Source: CAD feature listing. Evaluate the final solid. Frame: model axes, mm. A direction names the side the tool comes from. Round coordinates to 2 decimals unless told otherwise and drop trailing zeros. Order: outer loops, then holes, each group sorted by start corner. A loop starts at its lowest first (then second) coordinate and runs counter-clockwise, first axis right, second up. Notation, with made-up numbers: M 55.25,-4.75 L 100.25,-4.75 A25 ccw 100.25,34.25 Z; hole C 42.25,27.25 d10. An arc over 180 degrees is marked long. Use CSV: the item, a comma, the result in double quotes. Start each with the question number.
```python
from build123d import *

# Parameters (mm, degrees)
IZIM1_R                     = 2.35
IZIM1_R_2                   = 0.5
Y_KSEKLIK_EKSTR_ZYON1_DEPTH = 1.5
IZIM1_3_R                   = 2.35
IZIM1_3_R_2                 = 1.275
Y_KSEKLIK_EKSTR_ZYON2_DEPTH = 0.5
IZIM2_R                     = 3.45
IZIM2_R_2                   = 2.3
Y_KSEKLIK_EKSTR_ZYON3_DEPTH = 2.5
RADYUS1_R                   = 0.1


with BuildPart() as part:
    # izim1 → Y_kseklik-Ekstr_zyon1 (new body)
    with BuildSketch(Plane(origin=(0, 0, 0), x_dir=(1, 0, 0), z_dir=(0, 1, 0))):
        with BuildLine():
            Line((1.9, 2.9), (1.9, 6.05))
            ThreePointArc((1.9, 6.05), (0, 7.95), (-1.9, 6.05))
            Line((-1.9, 6.05), (-1.9, 3.45))
            Line((-1.9, 3.45), (-17.141537347, 1.487720889))
            ThreePointArc((-17.141537347, 1.487720889), (-18.45, 0), (-17.141537347, -1.487720889))
            Line((-17.141537347, -1.487720889), (-1.9, -3.45))
            Line((-1.9, -3.45), (-1.9, -6.75))
            ThreePointArc((-1.9, -6.75), (0, -8.65), (1.9, -6.75))
            Line((1.9, -6.75), (1.9, -2.9))
            Line((1.9, -2.9), (14.516515169, -1.490728915))
            ThreePointArc((14.516515169, -1.490728915), (15.85, 0), (14.516515169, 1.490728915))
            Line((14.516515169, 1.490728915), (1.9, 2.9))
        make_face()
        Circle(IZIM1_R, mode=Mode.SUBTRACT)
        with Locations((-16.95, 0)):
            Circle(IZIM1_R_2, mode=Mode.SUBTRACT)
        with Locations((-14.95, 0)):
            Circle(IZIM1_R_2, mode=Mode.SUBTRACT)
        with Locations((-12.95, 0)):
            Circle(IZIM1_R_2, mode=Mode.SUBTRACT)
        with Locations((-10.95, 0)):
            Circle(IZIM1_R_2, mode=Mode.SUBTRACT)
        with Locations((-8.95, 0)):
            Circle(IZIM1_R_2, mode=Mode.SUBTRACT)
        with Locations((-6.95, 0)):
            Circle(IZIM1_R_2, mode=Mode.SUBTRACT)
        with Locations((-4.95, 0)):
            Circle(IZIM1_R_2, mode=Mode.SUBTRACT)
        with Locations((14.35, 0)):
            Circle(IZIM1_R_2, mode=Mode.SUBTRACT)
        with Locations((12.35, 0)):
            Circle(IZIM1_R_2, mode=Mode.SUBTRACT)
        with Locations((10.35, 0)):
            Circle(IZIM1_R_2, mode=Mode.SUBTRACT)
        with Locations((8.35, 0)):
            Circle(IZIM1_R_2, mode=Mode.SUBTRACT)
        with Locations((6.35, 0)):
            Circle(IZIM1_R_2, mode=Mode.SUBTRACT)
        with Locations((4.35, 0)):
            Circle(IZIM1_R_2, mode=Mode.SUBTRACT)
        with Locations((0, 6.35)):
            Circle(IZIM1_R_2, mode=Mode.SUBTRACT)
        with Locations((0, 4.35)):
            Circle(IZIM1_R_2, mode=Mode.SUBTRACT)
        with Locations((0, -6.6)):
            Circle(IZIM1_R_2, mode=Mode.SUBTRACT)
        with Locations((0, -4.6)):
            Circle(IZIM1_R_2, mode=Mode.SUBTRACT)
    extrude(amount=Y_KSEKLIK_EKSTR_ZYON1_DEPTH)

    # izim1_3 → Y_kseklik-Ekstr_zyon2 (add)
    with BuildSketch(Plane(origin=(0, 0, 0), x_dir=(1, 0, 0), z_dir=(0, 1, 0))):
        Circle(IZIM1_3_R)
        Circle(IZIM1_3_R_2, mode=Mode.SUBTRACT)
    extrude(amount=Y_KSEKLIK_EKSTR_ZYON2_DEPTH)

    # izim2 → Y_kseklik-Ekstr_zyon3 (add)
    with BuildSketch(Plane.XZ):
        Circle(IZIM2_R)
        Circle(IZIM2_R_2, mode=Mode.SUBTRACT)
    extrude(amount=Y_KSEKLIK_EKSTR_ZYON3_DEPTH)

    # Radyus1
    radyus1_edges = [part.edges().sort_by_distance(p)[0] for p in [
        (1.9, 0.75, -2.9),
        (1.9, 0.75, 2.9),
        (-1.9, 0.75, 3.45),
        (-1.9, 0.75, -3.45),
    ]]
    fillet(radyus1_edges, radius=RADYUS1_R)


solid = part.part
```
(1) Reachability of faces 4 (the face through (-1.825, -1.232, -1.4)), 5 (the face through (7.85, 0.74, -0.02)), 6 (the face through (1.01, 0.5, 1.01)) from +Z, -Z, +X, -X, +Y, -Y: full face, straight path, thin tool, end or side. Return the list, or none.
(2) Section B-B on x = -12.95. Return loops of the section in (y, z), plus the area to 3 significant figures.
(3) Line query: line 1 along Z through (x, y) = (0, 1.2); line 2 along Y through (x, z) = (9, -0.75); line 3 along Z through (x, y) = (0, -0.05). Output: solid intervals per line, ascending.
(4) Section A-A on z = -4.35. Return loops of the section in (x, y), plus the area to 3 significant figures.
(5) Contact query for flat-ended pins moving along their axis: P1, Ø3, axis at x = 12, z = -4.5, coming from the +Y side; P2, Ø1.6, axis at y = 0.5, z = -5.5, coming from the -X side; P3, Ø2, axis at x = 1, y = -0.5, coming from the +Z side; P4, Ø3.5, axis at x = 0, z = 0, coming from the -Y side. Output: stop coordinate, or through.
(6) Section C-C on z = 0. Give the number of separate pieces and of enclosed holes in the cut face, plus the area to 3 significant figures.
(7) Draft query along X for faces 1 (the face through (0.231, 0.74, 7.044)), 2 (the face through (8.34, 0.74, -2.18)), 3 (the face through (-1.9, 1, -5)). Return one class per face: pulls with the +X half, pulls with the -X half, needs draft (parallel to the pull), parting line crosses it, or undercut.
(8) Section D-D on z = 7.5. Return loops of the section in (x, y), plus the area to 3 significant figures.
Results below:
1,face 4,"-Y"
1,face 5,"+Y, -Y"
1,face 6,"+Y"
2,outline,"M 0,-2.03 L 1.5,-2.03 L 1.5,-0.5 L 0,-0.5 Z; M 0,0.5 L 1.5,0.5 L 1.5,2.03 L 0,2.03 Z"
2,area,"4.58 mm2"
3,line 1,"z = -7.95 to -6.85, -5.85 to -4.85, -3.85 to -2.35, 2.35 to 4.1, 5.1 to 6.1, 7.1 to 8.65"
3,line 2,"y = 0 to 1.5"
3,line 3,"z = -3.45 to -2.3, 2.3 to 3.45"
4,outline,"M -1.9,0 L -0.5,0 L -0.5,1.5 L -1.9,1.5 Z; M 0.5,0 L 1.9,0 L 1.9,1.5 L 0.5,1.5 Z"
4,area,"4.20 mm2"
5,P1,"passes through"
5,P2,"stops at x = -1.9"
5,P3,"stops at z = 8.65"
5,P4,"stops at y = 0"
6,separate pieces,"15"
6,enclosed holes,"0"
6,area,"31.7 mm2"
7,face 1,"undercut"
7,face 2,"pulls with the +X half"
7,face 3,"pulls with the -X half"
8,outline,"M -1.75,0 L 1.75,0 L 1.75,1.5 L -1.75,1.5 Z"
8,area,"5.24 mm2"
